from build123d import *

# Parameters (mm, degrees)
SKETCH016_W             = 30
SKETCH016_H             = 13
PAD006_DEPTH            = 11
GROOVE001_ANGLE         = 180
SKETCH018_R             = 1.5
POCKET007_DEPTH         = 20
SKETCH019_R             = 3.5
POCKET008_DEPTH         = 3
SKETCH041_R             = 2.5
POCKET017_DEPTH         = 3
BODY001_PLACEMENT_ANGLE = 180


with BuildPart() as part:
    # Sketch016 → Pad006 (new body)
    with BuildSketch(Plane.XY):
        with Locations((-25, 6.5)):
            Rectangle(SKETCH016_W, SKETCH016_H)
    extrude(amount=PAD006_DEPTH)

    # Sketch017 (on Face5 of Pad006) → Groove001 (revolve, cut)
    with BuildSketch(Plane(origin=(0, 0, 0), x_dir=(1, 0, 0), z_dir=(0, 0, -1))):
        Polygon((-33, -13), (-33, -10.65), (-31.03, -10.65), (-31.03, -4.35), (-33, -4.35), (-33, 0), (-25, 0), (-25, -13), align=None)
    revolve(axis=Axis((-25, 0, 0), (0, 1, 0)), revolution_arc=GROOVE001_ANGLE, mode=Mode.SUBTRACT)

    # Sketch018 (on Face6 of Groove001) → Pocket007 (cut)
    with BuildSketch(Plane.XY.offset(11)):
        with Locations((-36.5, 6.5)):
            Circle(SKETCH018_R)
        with Locations((-13.5, 6.5)):
            Circle(SKETCH018_R)
    extrude(amount=-POCKET007_DEPTH, mode=Mode.SUBTRACT)

    # Sketch019 (on Face6 of Pocket007) → Pocket008 (cut)
    with BuildSketch(Plane.XY.offset(11)):
        with Locations((-36.5, 6.5)):
            Circle(SKETCH019_R)
        with Locations((-13.5, 6.5)):
            Circle(SKETCH019_R)
    extrude(amount=-POCKET008_DEPTH, mode=Mode.SUBTRACT)

    # Sketch041 (on Face6 of Pocket008) → Pocket017 (cut)
    with BuildSketch(Plane.XY.offset(11)):
        with Locations((-20.75, 4)):
            Circle(SKETCH041_R)
    extrude(amount=-POCKET017_DEPTH, mode=Mode.SUBTRACT)


with BuildPart() as part_1:
    # Body001 placement: moved
    add(part.part.moved(Location((-10, 0, -11))).rotate(Axis((-10, 0, -11), (0, 1, 0)), BODY001_PLACEMENT_ANGLE))


solid = part_1.part
CAD build for the part. Positions are in the model's coordinates, mm. A direction names the side the tool comes from. Coordinates: 2 decimals unless noted, no trailing zeros. Write each loop counter-clockwise with the first axis right and the second up, starting at its lowest first coordinate (ties: lowest second). Pieces come first, ordered by that corner, then holes. Notation, with made-up numbers: M 69,34 L 91,34 A19 ccw 91,50 Z; hole C 63.5,22.5 d8. An arc over 180 degrees is marked long. Return JSON: item names as keys, results as strings.
Item 1: Slice it at D-D, the plane z = -18.5. Write the cut outline in (x, y).
Findings below:
{"outline": "M 0,0 L 12.22,0 L 12.22,4.35 L 17.78,4.35 L 17.78,0 L 30,0 L 30,13 L 17.78,13 L 17.78,10.65 L 12.22,10.65 L 12.22,13 L 0,13 Z; hole C 3.5,6.5 d3; hole C 26.5,6.5 d3"}
Item 2: Slice it at B-B, the plane z = -15.5. Write the cut outline in (x, y), and give its area (3 significant figures).
Findings below:
{"outline": "M 0,0 L 8.39,0 L 8.39,4.35 L 10.99,4.35 L 10.99,10.65 L 8.39,10.65 L 8.39,13 L 0,13 Z; M 19.01,4.35 L 21.61,4.35 L 21.61,0 L 30,0 L 30,13 L 21.61,13 L 21.61,10.65 L 19.01,10.65 Z; hole C 3.5,6.5 d3; hole C 26.5,6.5 d3", "area": "237 mm2"}
Item 3: Drop flat-ended pins along their axis: pin 1 Ø4 at (x, y) = (3.5, 6.5) entering from -Z; pin 2 Ø4 at (x, z) = (17, -16) entering from +Y; pin 3 Ø1.8 at (x, y) = (3.5, 6.5) entering from -Z. Give the stop position or say it passes through.
Findings below:
{"pin 1": "stops at z = -19", "pin 2": "stops at y = 10.65", "pin 3": "passes through"}
Item 4: Two-plate mould, pull along X, no slides. Class faces 5 (the flat face through (0, 6, -16)), 6 (the flat face through (15, 0, -20)), 7 (the cylindrical face through (15, 12, -19)): +X half, -X half, draft (parallel to the pull), parting line (faces both ways), or undercut.
Findings below:
{"face 5": "-X half", "face 6": "draft", "face 7": "undercut"}
Item 5: Which spindle directions (+Z, -Z, +X, -X, +Y, -Y) get a long thin tool onto all of the face, cutting with end or side? Do faces 1 (the flat face through (30, 6, -16)), 2 (the flat face through (2.8, 5, -19)), 3 (the flat face through (15, 10.65, -17.4)), 4 (the cylindrical face through (15, 2, -19)). Say none if no direction does.
Findings below:
{"face 1": "+Z, -Z, +X, +Y, -Y", "face 2": "-Z", "face 3": "+Z, +Y", "face 4": "+Z, -Y"}
Item 6: Slice it at C-C, the plane x = 15. Write the cut outline in (y, z).
Findings below:
{"outline": "M 0,-22 L 13,-22 L 13,-19 L 10.65,-19 L 10.65,-17.03 L 4.35,-17.03 L 4.35,-19 L 0,-19 Z"}
Item 7: Probe line 1 (Y direction, x = 3.5, z = -21.25); line 2 (Y direction, x = 3.5, z = -14.5); line 3 (X direction, y = 4.25, z = -19.25). List the from-to ranges inside material, lowest first. Write a range as from..to.
Findings below:
{"line 1": "y = 0..3, 10..13", "line 2": "y = 0..5, 8..13", "line 3": "x = 0..0.82, 6.18..8.26, 13.24..23.82, 29.18..30"}
